Work out the finished part from the listing and answer in its coordinate system (mm). A direction names the side the tool comes from. Coordinates: 2 decimals unless noted, no trailing zeros. Loops run counter-clockwise (first coordinate to the right, second up) from the corner with the lowest first, then second, coordinate; pieces in that order, holes last. Notation, with made-up numbers: (78, 61.5) -> (103, 61.5) arc R17 cw to (103, 72.5) -> close; hole circle Ø2 at (-29, -20.75). An arc over 180 degrees is marked (long way). Use a Markdown table: item, result. Add a question column.
```python
from build123d import *

# Parameters (mm, degrees)
ESQUISSE1_W             = 8.382
ESQUISSE1_H             = 2.54
BOSS_EXTRU_1_DEPTH      = 1.905
ESQUISSE2_W             = 0.635
ESQUISSE2_H             = 2.54
BOSS_EXTRU_2_DEPTH      = 0.508
ESQUISSE3_W             = 0.762
ESQUISSE3_H             = 0.762
BOSS_EXTRU_3_DEPTH      = 0.508
ESQUISSE4_W             = 1.905
ESQUISSE4_H             = 2.54
BOSS_EXTRU_4_DEPTH      = 2.286
ESQUISSE5_W             = 2.54
ESQUISSE5_H             = 11.176
BOSS_EXTRU_5_DEPTH      = 0.635
ESQUISSE6_R             = 0.538815367
BOSS_EXTRU_6_DEPTH      = 0.254
ESQUISSE7_W             = 0.762
ESQUISSE7_H             = 0.762
BOSS_EXTRU_7_DEPTH      = 12.446
ENL_V_MAT_EXTRU_1_DEPTH = 2.54
ENL_V_MAT_EXTRU_2_DEPTH = 2.54
ENL_V_MAT_EXTRU_3_DEPTH = 2.54
ENL_V_MAT_EXTRU_4_DEPTH = 2.54
ESQUISSE12_W            = 0.762
ESQUISSE12_H            = 0.762
ENL_V_MAT_EXTRU_5_DEPTH = 7.62
CHANFREIN1_SIZE         = 0.254
CHANFREIN2_SIZE         = 0.381


with BuildPart() as part:
    # Esquisse1 → Boss.-Extru.1 (new body)
    with BuildSketch(Plane(origin=(-1.27, 0, 0), x_dir=(0, -1, 0), z_dir=(-1, 0, 0))):
        with Locations((-6.985, 0)):
            Rectangle(ESQUISSE1_W, ESQUISSE1_H)
    extrude(amount=-BOSS_EXTRU_1_DEPTH)

    # Esquisse2 → Boss.-Extru.2 (add)
    with BuildSketch(Plane.XZ.offset(-2.794)):
        with Locations((-0.9525, 0)):
            Rectangle(ESQUISSE2_W, ESQUISSE2_H)
    extrude(amount=BOSS_EXTRU_2_DEPTH)

    # Esquisse3 → Boss.-Extru.3 (add)
    with BuildSketch(Plane.XZ.offset(-2.794)):
        Rectangle(ESQUISSE3_W, ESQUISSE3_H)
    extrude(amount=BOSS_EXTRU_3_DEPTH)

    # Esquisse4 → Boss.-Extru.4 (add)
    with BuildSketch(Plane.XZ.offset(-2.286)):
        with Locations((-0.3175, 0)):
            Rectangle(ESQUISSE4_W, ESQUISSE4_H)
    extrude(amount=BOSS_EXTRU_4_DEPTH)

    # Esquisse5 → Boss.-Extru.5 (add)
    with BuildSketch(Plane(origin=(0.635, 0, 0), x_dir=(0, 0, -1), z_dir=(1, 0, 0))):
        with Locations((0, 5.588)):
            Rectangle(ESQUISSE5_W, ESQUISSE5_H)
    extrude(amount=BOSS_EXTRU_5_DEPTH)

    # Esquisse6 → Boss.-Extru.6 (add)
    with BuildSketch(Plane.XZ):
        with Locations(Location((0, 0, 0), (0, 0, 90))):
            Circle(ESQUISSE6_R)
    extrude(amount=BOSS_EXTRU_6_DEPTH)

    # Esquisse7 → Boss.-Extru.7 (add)
    with BuildSketch(Plane.XZ.offset(0.254)):
        Rectangle(ESQUISSE7_W, ESQUISSE7_H)
    extrude(amount=BOSS_EXTRU_7_DEPTH)

    # Esquisse8 → Enlèv. mat.-Extru.1 (cut)
    with BuildSketch(Plane.XZ):
        Polygon((-1.27, 1.27), (-1.27, 0.889), (-0.889, 1.27), align=None)
    extrude(amount=-ENL_V_MAT_EXTRU_1_DEPTH, mode=Mode.SUBTRACT)

    # Esquisse9 → Enlèv. mat.-Extru.2 (cut)
    with BuildSketch(Plane.XZ):
        Polygon((-1.27, -1.27), (-0.889, -1.27), (-1.27, -0.889), align=None)
    extrude(amount=-ENL_V_MAT_EXTRU_2_DEPTH, mode=Mode.SUBTRACT)

    # Esquisse10 → Enlèv. mat.-Extru.3 (cut)
    with BuildSketch(Plane.XZ):
        Polygon((1.27, 1.27), (0.889, 1.27), (1.27, 0.889), align=None)
    extrude(amount=-ENL_V_MAT_EXTRU_3_DEPTH, mode=Mode.SUBTRACT)

    # Esquisse11 → Enlèv. mat.-Extru.4 (cut)
    with BuildSketch(Plane.XZ):
        Polygon((1.27, -1.27), (1.27, -0.889), (0.889, -1.27), align=None)
    extrude(amount=-ENL_V_MAT_EXTRU_4_DEPTH, mode=Mode.SUBTRACT)

    # Esquisse12 → Enlèv. mat.-Extru.5 (cut)
    with BuildSketch(Plane(origin=(0, 11.176, 0), x_dir=(-1, 0, 0), z_dir=(0, 1, 0))):
        Rectangle(ESQUISSE12_W, ESQUISSE12_H)
    extrude(amount=-ENL_V_MAT_EXTRU_5_DEPTH, mode=Mode.SUBTRACT)

    # Chanfrein1
    chanfrein1_edges = [part.edges().sort_by_distance(p)[0] for p in [
        (0.381, -12.7, 0),
        (0, -12.7, 0.381),
        (-0.381, -12.7, 0),
        (0, -12.7, -0.381),
    ]]
    chamfer(chanfrein1_edges, length=CHANFREIN1_SIZE)

    # Chanfrein2
    chanfrein2_edges = [part.edges().sort_by_distance(p)[0] for p in [
        (0, 11.176, 0.381),
        (0.381, 11.176, 0),
        (0, 11.176, -0.381),
        (-0.381, 11.176, 0),
    ]]
    chamfer(chanfrein2_edges, length=CHANFREIN2_SIZE)


solid = part.part
```
Item 1: For faces 1 (the face through (0, 0, -1)), 2 (the face through (-1, 11.176, 0)), determine the directions among +Z, -Z, +X, -X, +Y, -Y from which every point of the face is accessible in a straight line to the end or side of a thin tool.
Item 2: Section A-A (y = 6.25) is taken. Determine the outline of the cut face in (x, z), then the cut area to 3 significant figures.
Item 3: Given pin 1 (0.6 mm diameter, centred on y = -5, z = 0, fed in from +X); pin 2 (1.5 mm diameter, centred on x = 0, y = -7.5, fed in from -Z), each flat-ended and moving along its own axis, determine where each tip first touches the part or whether it passes through.
Item 4: Find the intervals of material crossed by probe 1 along Z at (x, y) = (-0.25, 5); probe 2 along Y at (x, z) = (-0.55, 0.95); probe 3 along Y at (x, z) = (-0.85, 0.85), in increasing order.
Item 5: Section B-B (y = 0.75) is taken. Determine the outline of the cut face in (x, z), then the cut area to 3 significant figures.
Item 6: Section C-C (y = -10.25) is taken. Determine the outline of the cut face in (x, z), then the cut area to 3 significant figures.
Output:
| question | item | result |
|---|---|---|
| 1 | face 1 | -Y |
| 1 | face 2 | +Z, -Z, +X, -X, +Y |
| 2 | outline | (-1.27, -1.27) -> (1.27, -1.27) -> (1.27, 1.27) -> (-1.27, 1.27) -> close; hole (-0.38, -0.38) -> (0.38, -0.38) -> (0.38, 0.38) -> (-0.38, 0.38) -> close |
| 2 | area | 5.87 mm2 |
| 3 | pin 1 | stops at x = 0.38 |
| 3 | pin 2 | stops at z = -0.38 |
| 4 | probe 1 | z = -1.27 to -0.38, 0.38 to 1.27 |
| 4 | probe 2 | y = 0 to 2.29, 2.79 to 11.18 |
| 4 | probe 3 | y = 0 to 11.18 |
| 5 | outline | (-1.27, -0.89) -> (-0.89, -1.27) -> (0.89, -1.27) -> (1.27, -0.89) -> (1.27, 0.89) -> (0.89, 1.27) -> (-0.89, 1.27) -> (-1.27, 0.89) -> close |
| 5 | area | 6.16 mm2 |
| 6 | outline | (-0.38, -0.38) -> (0.38, -0.38) -> (0.38, 0.38) -> (-0.38, 0.38) -> close |
| 6 | area | 0.581 mm2 |
